```python
from build123d import *

# Parameters (mm, degrees)
SKETCH4_W                = 120
SKETCH4_H                = 84
BOSS_EXTRUDE2_DEPTH      = 50
BOSS_EXTRUDE4_DEPTH      = 48
BOSS_EXTRUDE4_DEPTH_BACK = 5.717293385
SKETCH5_W                = 116
SKETCH5_H                = 67
FILLET2_R                = 2
FILLET3_R                = 2


# Some blends are built 0.0001 mm under size
with BuildPart() as part:
    # Sketch4 → Boss-Extrude2 (new body)
    with BuildSketch(Plane(origin=(0, 0, 0), x_dir=(1, 0, 0), z_dir=(0, 1, 0))):
        with Locations((60, 42)):
            Rectangle(SKETCH4_W, SKETCH4_H)
    extrude(amount=BOSS_EXTRUDE2_DEPTH)


with BuildPart() as body_2:
    # Sketch5 → Boss-Extrude4 (new, two sides: drawn at the far end of the back side and taken through both)
    with BuildSketch(Plane(origin=(0, 0, 0), x_dir=(1, 0, 0), z_dir=(0, 1, 0)).offset(-BOSS_EXTRUDE4_DEPTH_BACK)):
        with Locations((60, 35.5)):
            Rectangle(SKETCH5_W, SKETCH5_H)
    extrude(amount=BOSS_EXTRUDE4_DEPTH + BOSS_EXTRUDE4_DEPTH_BACK)


with BuildPart() as part_1:
    add(part.part)

    # Combine1: cut body 2
    add(body_2.part, mode=Mode.SUBTRACT)

    # Fillet2
    fillet2_edges = [part_1.edges().sort_by_distance(p)[0] for p in [
        (0, 0, -42),
        (60, 0, -84),
        (120, 0, -42),
        (60, 0, 0),
    ]]
    fillet(fillet2_edges, radius=FILLET2_R - 0.0001)  # a hair under: the kernel refuses the full size

    # Fillet3
    # the kernel refuses this fillet: 2 mm, written as the material it takes off along each edge
    with BuildSketch(Plane(origin=(118, 0, -2), x_dir=(1, 0, 0), z_dir=(0, 0, -1))) as fillet3_piece_1:
        with BuildLine():
            CenterArc((0.0001, -1.9999), 1.9999, 0, 90)
            Line((2, -1.9999), (2, 0))
            Line((2, 0), (0.0001, 0))
        make_face()
    revolve(axis=Axis((118, 0, -2), (0, -1, 0)), revolution_arc=90, mode=Mode.SUBTRACT)
    with BuildSketch(Plane(origin=(118, 0, -82), x_dir=(0, 0, -1), z_dir=(-1, 0, 0))) as fillet3_piece_2:
        with BuildLine():
            CenterArc((0.0001, -1.9999), 1.9999, 0, 90)
            Line((2, -1.9999), (2, 0))
            Line((2, 0), (0.0001, 0))
        make_face()
    revolve(axis=Axis((118, 0, -82), (0, -1, 0)), revolution_arc=90, mode=Mode.SUBTRACT)
    with BuildSketch(Plane(origin=(2, 0, -2), x_dir=(0, 0, 1), z_dir=(1, 0, 0))) as fillet3_piece_3:
        with BuildLine():
            CenterArc((0.0001, -1.9999), 1.9999, 0, 90)
            Line((2, -1.9999), (2, 0))
            Line((2, 0), (0.0001, 0))
        make_face()
    revolve(axis=Axis((2, 0, -2), (0, -1, 0)), revolution_arc=90, mode=Mode.SUBTRACT)
    with BuildSketch(Plane(origin=(2, 0, -82), x_dir=(-1, 0, 0), z_dir=(0, 0, 1))) as fillet3_piece_4:
        with BuildLine():
            CenterArc((0.0001, -1.9999), 1.9999, 0, 90)
            Line((2, -1.9999), (2, 0))
            Line((2, 0), (0.0001, 0))
        make_face()
    revolve(axis=Axis((2, 0, -82), (0, -1, 0)), revolution_arc=90, mode=Mode.SUBTRACT)
    with BuildSketch(Plane(origin=(118, 48, -82), x_dir=(1, 0, 0), z_dir=(0, 1, 0))) as fillet3_piece_5_section:
        Polygon((0, 0), (FILLET3_R, 0), (FILLET3_R, FILLET3_R), (0, FILLET3_R), align=None)
    fillet3_piece_5 = extrude(amount=FILLET3_R, mode=Mode.PRIVATE)
    fillet3_piece_5 = fillet3_piece_5 - Plane(origin=(118, 48, -82), x_dir=(-0.7071067811865475, 0, 0.7071067811865475), z_dir=(0, 1, 0)) * Sphere(FILLET3_R, mode=Mode.PRIVATE)
    add(fillet3_piece_5, mode=Mode.SUBTRACT)
    with BuildSketch(Plane(origin=(2, 48, -82), x_dir=(0, 1, 0), z_dir=(-1, 0, 0))) as fillet3_piece_6_section:
        Polygon((0, 0), (FILLET3_R, 0), (FILLET3_R, FILLET3_R), (0, FILLET3_R), align=None)
    fillet3_piece_6 = extrude(amount=FILLET3_R, mode=Mode.PRIVATE)
    fillet3_piece_6 = fillet3_piece_6 - Plane(origin=(2, 48, -82), x_dir=(0, -0.7071067811865475, 0.7071067811865475), z_dir=(-1, 0, 0)) * Sphere(FILLET3_R, mode=Mode.PRIVATE)
    add(fillet3_piece_6, mode=Mode.SUBTRACT)
    with BuildSketch(Plane(origin=(2, 48, -2), x_dir=(-1, 0, 0), z_dir=(0, 0, 1))) as fillet3_piece_7_section:
        Polygon((0, 0), (FILLET3_R, 0), (FILLET3_R, -FILLET3_R), (0, -FILLET3_R), align=None)
    fillet3_piece_7 = extrude(amount=FILLET3_R, mode=Mode.PRIVATE)
    fillet3_piece_7 = fillet3_piece_7 - Plane(origin=(2, 48, -2), x_dir=(0.7071067811865475, -0.7071067811865475, 0), z_dir=(0, 0, 1)) * Sphere(FILLET3_R, mode=Mode.PRIVATE)
    add(fillet3_piece_7, mode=Mode.SUBTRACT)
    with BuildSketch(Plane(origin=(118, 48, -2), x_dir=(0, 1, 0), z_dir=(0, 0, 1))) as fillet3_piece_8_section:
        Polygon((0, 0), (FILLET3_R, 0), (FILLET3_R, -FILLET3_R), (0, -FILLET3_R), align=None)
    fillet3_piece_8 = extrude(amount=FILLET3_R, mode=Mode.PRIVATE)
    fillet3_piece_8 = fillet3_piece_8 - Plane(origin=(118, 48, -2), x_dir=(-0.7071067811865475, -0.7071067811865475, 0), z_dir=(0, 0, 1)) * Sphere(FILLET3_R, mode=Mode.PRIVATE)
    add(fillet3_piece_8, mode=Mode.SUBTRACT)
    with BuildSketch(Plane(origin=(118, 50, -84), x_dir=(0, 0, 1), z_dir=(-1, 0, 0))) as fillet3_piece_9:
        with BuildLine():
            CenterArc((FILLET3_R, -FILLET3_R), FILLET3_R, 90, 90)
            Line((0, -FILLET3_R), (0, 0))
            Line((0, 0), (FILLET3_R, 0))
        make_face()
    extrude(amount=116, mode=Mode.SUBTRACT)
    with BuildSketch(Plane(origin=(0, 50, -82), x_dir=(0, -1, 0), z_dir=(0, 0, 1))) as fillet3_piece_10:
        with BuildLine():
            CenterArc((FILLET3_R, FILLET3_R), FILLET3_R, 180, 90)
            Line((0, FILLET3_R), (0, 0))
            Line((0, 0), (FILLET3_R, 0))
        make_face()
    extrude(amount=80, mode=Mode.SUBTRACT)
    with BuildSketch(Plane(origin=(2, 50, 0), x_dir=(0, -1, 0), z_dir=(1, 0, 0))) as fillet3_piece_11:
        with BuildLine():
            CenterArc((FILLET3_R, FILLET3_R), FILLET3_R, 180, 90)
            Line((0, FILLET3_R), (0, 0))
            Line((0, 0), (FILLET3_R, 0))
        make_face()
    extrude(amount=116, mode=Mode.SUBTRACT)
    with BuildSketch(Plane(origin=(0, 0, 0), x_dir=(1, 0, 0), z_dir=(0, 1, 0)), Plane(origin=(0, 0, -84), x_dir=(0, 0, 1), z_dir=(0, 1, 0))) as fillet3_piece_12:
        with BuildLine():
            CenterArc((FILLET3_R, FILLET3_R), FILLET3_R, 180, 90)
            Line((0, FILLET3_R), (0, 0))
            Line((0, 0), (FILLET3_R, 0))
        make_face()
    extrude(amount=48, mode=Mode.SUBTRACT)
    with BuildSketch(Plane(origin=(120, 0, -84), x_dir=(0, 0, 1), z_dir=(0, 1, 0)), Plane(origin=(120, 0, 0), x_dir=(-1, 0, 0), z_dir=(0, 1, 0))) as fillet3_piece_13:
        with BuildLine():
            CenterArc((FILLET3_R, -FILLET3_R), FILLET3_R, 90, 90)
            Line((0, -FILLET3_R), (0, 0))
            Line((0, 0), (FILLET3_R, 0))
        make_face()
    extrude(amount=48, mode=Mode.SUBTRACT)
    with BuildSketch(Plane(origin=(120, 50, -2), x_dir=(-1, 0, 0), z_dir=(0, 0, -1))) as fillet3_piece_14:
        with BuildLine():
            CenterArc((FILLET3_R, -FILLET3_R), FILLET3_R, 90, 90)
            Line((0, -FILLET3_R), (0, 0))
            Line((0, 0), (FILLET3_R, 0))
        make_face()
    extrude(amount=80, mode=Mode.SUBTRACT)


solid = part_1.part
```
CAD build for the part. Positions are in the model's coordinates, mm. A direction names the side the tool comes from. Coordinates: 2 decimals unless noted, no trailing zeros. Order: outer loops, then holes, each group sorted by start corner. A loop starts at its lowest first (then second) coordinate and runs counter-clockwise, first axis right, second up.
(1) Mould opens along X. For faces 3 (the face through (59, 24, -69)), 4 (the face through (118, 24, -35)), 5 (the face through (0, 25, -41)), 6 (the face through (60, 0, -78)) say: released by +X, released by -X, zero draft, split by the parting line, or undercut.
Solution:
face 3: undercut
face 4: undercut
face 5: released by -X
face 6: zero draft
(2) Drill centre lines: L1, parallel to X at y = 20.5, z = -22; L2, parallel to Z at x = 37, y = 40.5; L3, parallel to Y at x = 39.5, z = -32. Where is each one in solid material? Low to high.
Solution:
L1: x = 0 to 2, 118 to 120
L2: z = -84 to -69, -2 to 0
L3: y = 48 to 50
(3) Saw through at A-A, the plane y = 6.5. Write the cut outline in (x, z), and give its area (3 significant figures).
Solution:
outline: (0, -82) arc R2 ccw to (2, -84) - (118, -84) arc R2 ccw to (120, -82) - (120, -2) arc R2 ccw to (118, 0) - (2, 0) arc R2 ccw to (0, -2) - close; hole (2, -69) - (118, -69) - (118, -2) - (2, -2) - close
area: 2,300 mm2
(4) Which spindle directions (+Z, -Z, +X, -X, +Y, -Y) get a long thin tool onto all of the face, cutting with end or side? Do faces 1 (the face through (59, 48, -36)), 2 (the face through (59, 50, -43)). Say none if no direction does.
Solution:
face 1: -Y
face 2: +Z, -Z, +X, -X, +Y
